The listing builds one solid part. Answer for the finished solid, in the listing's coordinates (mm). A direction names the side the tool comes from. Coordinates: 2 decimals unless noted, no trailing zeros. Write each loop counter-clockwise with the first axis right and the second up, starting at its lowest first coordinate (ties: lowest second). Pieces come first, ordered by that corner, then holes.
from build123d import *

# Parameters (mm, degrees)
PAD_DEPTH       = 19
POCKET_DEPTH    = 7
POCKET001_DEPTH = 5
POCKET002_DEPTH = 3.5
POCKET003_DEPTH = 3.501
FILLET_R        = 0.5
FILLET001_R     = 0.5


with BuildPart() as part:
    # Sketch → Pad (new body)
    with BuildSketch(Plane(origin=(0, 0, 0), x_dir=(0, -1, 0), z_dir=(0, 0, 1))):
        with BuildLine():
            ThreePointArc((8.485307, -8.485256), (0, 12), (-8.485307, -8.485256))
            Line((-8.485307, -8.485256), (-4.970563, -12))
            Line((-4.970563, -12), (4.970563, -12))
            Line((4.970563, -12), (8.485307, -8.485256))
        make_face()
    extrude(amount=-PAD_DEPTH)

    # Sketch002 → Pocket (cut)
    with BuildSketch(Plane(origin=(0, 0, 0), x_dir=(0, -1, 0), z_dir=(0, 0, 1))):
        with BuildLine():
            ThreePointArc((-10.2, 0), (0, -10.2), (10.2, 0))
            Line((10.2, 20), (10.2, 0))
            Line((-10.2, 20), (10.2, 20))
            Line((-10.2, 0), (-10.2, 20))
        make_face()
    extrude(amount=-POCKET_DEPTH, mode=Mode.SUBTRACT)

    # Sketch003 → Pocket001 (cut)
    with BuildSketch(Plane(origin=(0, 0, -7), x_dir=(0, -1, 0), z_dir=(0, 0, 1))):
        with BuildLine():
            ThreePointArc((-7, 0), (-4.949747, -4.949747), (0, -7))
            Line((20, -7), (0, -7))
            Line((20, 20), (20, -7))
            Line((-7, 20), (20, 20))
            Line((-7, 0), (-7, 20))
        make_face()
    extrude(amount=-POCKET001_DEPTH, mode=Mode.SUBTRACT)

    # Sketch004 → Pocket002 (cut)
    with BuildSketch(Plane(origin=(0, 0, -12), x_dir=(0, -1, 0), z_dir=(0, 0, 1))):
        with BuildLine():
            ThreePointArc((-7.2, 0), (0, -7.2), (7.2, 0))
            Line((7.2, 20), (7.2, 0))
            Line((-7.2, 20), (7.2, 20))
            Line((-7.2, 0), (-7.2, 20))
        make_face()
    extrude(amount=-POCKET002_DEPTH, mode=Mode.SUBTRACT)

    # Sketch005 → Pocket003 (cut, through all)
    with BuildSketch(Plane(origin=(0, 0, -15.5), x_dir=(0, -1, 0), z_dir=(0, 0, 1))):
        with BuildLine():
            ThreePointArc((-3.5, -1e-06), (0, -3.5), (3.5, 0))
            Line((3.5, 20), (3.5, 0))
            Line((-3.5, 20), (3.5, 20))
            Line((-3.5, -1e-06), (-3.5, 20))
        make_face()
    extrude(amount=-POCKET003_DEPTH, mode=Mode.SUBTRACT)

    # Fillet
    fillet_edges = [part.edges().sort_by_distance(p)[0] for p in [
        (6.321392, -10.2, -3.5),
        (9.6, -7.2, -13.75),
        (11.47824, -3.5, -17.25),
        (11.47824, 3.5, -17.25),
        (9.6, 7.2, -13.75),
        (6.321392, 10.2, -3.5),
    ]]
    fillet(fillet_edges, radius=FILLET_R)

    # Fillet001
    fillet001_edges = [part.edges().sort_by_distance(p)[0] for p in [
        (9.746794, 7, -9.5),
    ]]
    fillet(fillet001_edges, radius=FILLET001_R)


solid = part.part
1. A tool of negligible diameter and unlimited length cuts with its end or side. For faces 1 (the flat face through (-7, -5, -9)), 2 (the cylindrical face through (-10.2, 0.2, -3.5)), 3 (the flat face through (5, 3.5, -17)), from which of +Z, -Z, +X, -X, +Y, -Y can it reach the whole face along a straight path? Write none if from no direction.
Results found:
face 1: +X, -Y
face 2: +Z, +X
face 3: +Z, -Z, +X
2. Flat-ended cylindrical pins translate along their axes: P1, Ø8, axis at x = 9, z = -15.5, coming from the +Y side; P2, Ø2, axis at x = 3.5, z = -7, coming from the -Y side; P3, Ø4, axis at x = 6.5, z = -13.5, coming from the +Y side. Find the tip coordinate at first contact, or state that the pin passes through.
Results found:
P1: stops at y = 10.91
P2: stops at y = -11.74
P3: stops at y = 11.12
3. Section D-D on x = 1 is taken. Give the vertices of the cut face in (y, z).
Results found:
outline: (-11.96, -19) - (-3.5, -19) - (-3.5, -15.5) - (-7.2, -15.5) - (-7.2, -12) - (-11.96, -12) - close; (-11.96, -7) - (-10.2, -7) - (-10.2, 0) - (-11.96, 0) - close; (3.5, -19) - (11.96, -19) - (11.96, 0) - (10.2, 0) - (10.2, -7) - (7, -7) - (7, -12) - (7.2, -12) - (7.2, -15.5) - (3.5, -15.5) - close
4. Section B-B on z = -16 is taken. Give the vertices of the cut face in (x, y).
Results found:
outline: (-12, -4.97) - (-8.49, -8.49) arc R12 ccw to (11.25, -4.17) arc R0.5 ccw to (10.78, -3.5) - (0, -3.5) arc R3.5 cw to (0, 3.5) - (10.78, 3.5) arc R0.5 ccw to (11.25, 4.17) arc R12 ccw to (-8.49, 8.49) - (-12, 4.97) - close
5. For a pull along Z with two mould halves and no side action, classify faces 4 (the cylindrical face through (-7.2, 0.16, -13.73)), 5 (the flat face through (-2.8, -2.5, -19)), 6 (the flat face through (2, -10.2, -3)) as pulls with the +Z half, pulls with the -Z half, needs draft (parallel to the pull), parting line crosses it, or undercut.
Results found:
face 4: undercut
face 5: pulls with the -Z half
face 6: needs draft
6. Section C-C on y = -5.75 is taken. Give the vertices of the cut face in (x, z), then the cut area to 3 significant figures.
Results found:
outline: (-11.22, -19) - (10.53, -19) - (10.53, -15.5) - (-4.33, -15.5) - (-4.33, -12) - (-7, -12) - (-7, -7) - (-8.42, -7) - (-8.42, 0) - (-11.22, 0) - close
area: 141 mm2
7. Find the intervals of material crossed by L1, parallel to Z at x = 3, y = -10.75; L2, parallel to Z at x = 5.5, y = -8; L3, parallel to Y at x = -0.25, z = -10.5, in increasing order.
Results found:
L1: z = -19 to -12, -7 to 0
L2: z = -19 to -12
L3: y = 7 to 12
8. Section A-A on x = -1.75 is taken. Give the vertices of the cut face in (y, z), then the cut area to 3 significant figures.
Results found:
outline: (-11.87, -19) - (-3.03, -19) - (-3.03, -15.5) - (-6.98, -15.5) - (-6.98, -12) - (-11.87, -12) - close; (-11.87, -7) - (-10.05, -7) - (-10.05, 0) - (-11.87, 0) - close; (3.03, -19) - (11.87, -19) - (11.87, 0) - (10.05, 0) - (10.05, -7) - (6.78, -7) - (6.78, -12) - (6.98, -12) - (6.98, -15.5) - (3.03, -15.5) - close
area: 147 mm2
